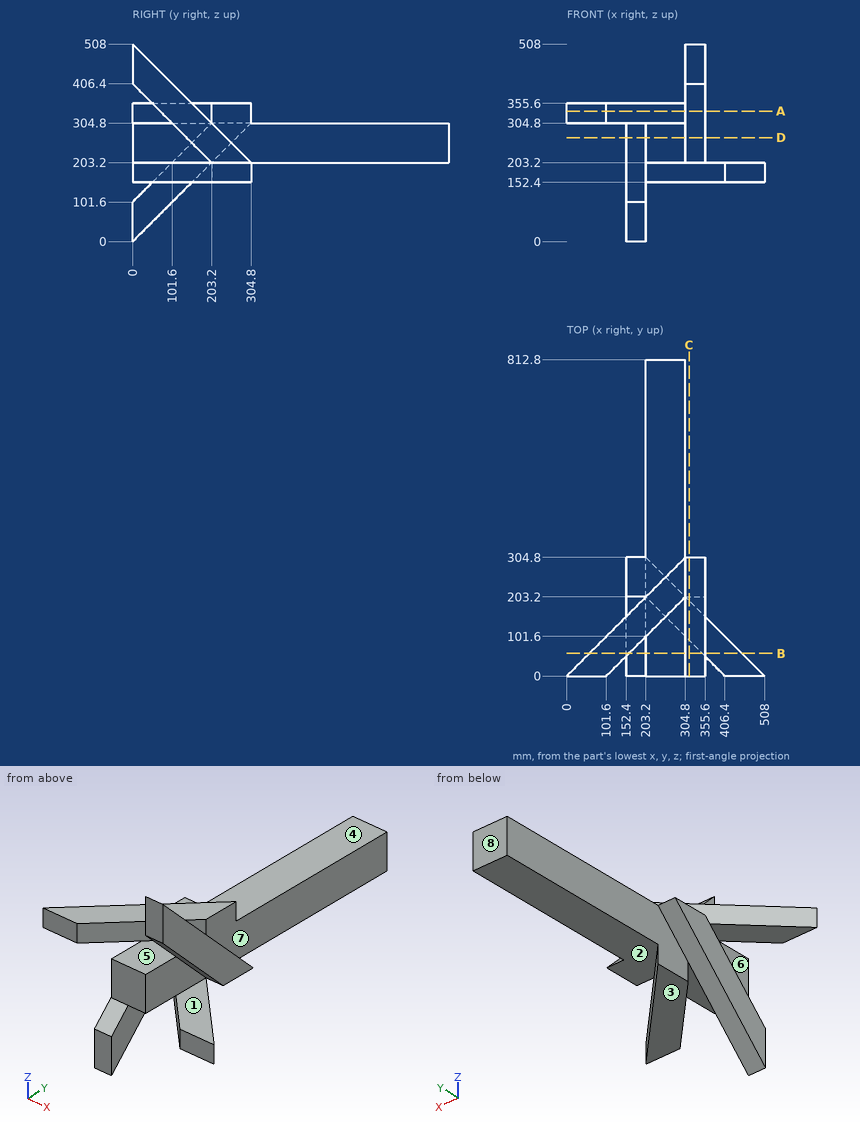
Check sheet for the drawn part. Datum: minimum x, y, z corner. Units: mm. A direction names the side the tool comes from. Coordinates: 2 decimals unless noted, no trailing zeros. Order: outer loops, then holes, each group sorted by start corner. A loop starts at its lowest first (then second) coordinate and runs counter-clockwise, first axis right, second up. Notation, with made-up numbers: (74, -35.75) -> (99, -35.75) arc R17 cw to (99, -23.75) -> close; hole circle Ø4 at (41.25, 72.5). An arc over 180 degrees is marked (long way). Write each question's results on one line, items separated by ' | '. Start each with the question number.
1) Section check B-B (y = 58). Enter the section's corners in (x, z).
2) Draft check along X on the marked faces 5, 6, 7 and 8. Enter one of: pulls with the +X half, pulls with the -X half, needs draft (parallel to the pull), parting line crosses it, or undercut.
3) Material ranges on line 1 along X through (y, z) = (584, 275); line 2 along Z through (x, y) = (405, 57), recorded low to high.
4) Depth check by flat-ended pin: pin 1 (4 mm diameter, centred on x = 352, z = 243, fed in from -Y); pin 2 (5 mm diameter, centred on y = 557.5, z = 208, fed in from -X); pin 3 (8 mm diameter, centred on y = 254.5, z = 186.5, fed in from +X). Enter the tip coordinate at first touch or a pass-through.
5) Section check A-A (z = 335.5). Enter the section's corners in (x, y), and give its area (3 significant figures).
6) Section check C-C (x = 314.5). Enter the section's corners in (y, z), and give its area (3 significant figures).
7) Section check D-D (z = 267.5). Enter the section's corners in (x, y).
8) Set-up check for the marked faces 1, 2, 3 and 4: record each of +Z, -Z, +X, -X, +Y, -Y from which the full face is reachable in a straight line by a thin tool's end or side.
Checked values:
1) outline: (58, 304.8) -> (159.6, 304.8) -> (159.6, 355.6) -> (58, 355.6) -> close; (152.4, 58) -> (203.2, 58) -> (203.2, 159.6) -> (152.4, 159.6) -> close; (203.2, 203.2) -> (304.8, 203.2) -> (304.8, 304.8) -> (203.2, 304.8) -> close; (304.8, 348.4) -> (355.6, 348.4) -> (355.6, 450) -> (304.8, 450) -> close; (348.4, 152.4) -> (450, 152.4) -> (450, 203.2) -> (348.4, 203.2) -> close
2) face 5: undercut | face 6: pulls with the -X half | face 7: pulls with the +X half | face 8: needs draft
3) line 1: 203.2 to 304.8 | line 2: 152.4 to 203.2
4) pin 1: y = 161.4 | pin 2: x = 203.2 | pin 3: x = 257.5
5) outline: (0, 0) -> (101.6, 0) -> (304.8, 203.2) -> (304.8, 304.8) -> close; (304.8, 70.9) -> (355.6, 70.9) -> (355.6, 172.5) -> (304.8, 172.5) -> close | area: 31,000 mm²
6) outline: (0, 406.4) -> (203.2, 203.2) -> (304.8, 203.2) -> (0, 508) -> close; (91.9, 152.4) -> (193.5, 152.4) -> (193.5, 203.2) -> (91.9, 203.2) -> close | area: 31,000 mm²
7) outline: (152.4, 165.9) -> (203.2, 165.9) -> (203.2, 0) -> (304.8, 0) -> (304.8, 138.9) -> (355.6, 138.9) -> (355.6, 240.5) -> (304.8, 240.5) -> (304.8, 812.8) -> (203.2, 812.8) -> (203.2, 267.5) -> (152.4, 267.5) -> close
8) face 1: +X, -Y | face 2: -Z, +X, +Y | face 3: -Z, +X, +Y, -Y | face 4: +Z, -X, +Y
